The listing builds one solid part. Answer for the finished solid, in the listing's coordinates (mm). Face numbers are marked on the shaded views. A direction names the side the tool comes from. Round coordinates to 2 decimals unless told otherwise and drop trailing zeros. Order: outer loops, then holes, each group sorted by start corner. A loop starts at its lowest first (then second) coordinate and runs counter-clockwise, first axis right, second up. Notation, with made-up numbers: (51, -16) -> (81, -16) arc R24 cw to (81, 16) -> close; hole circle Ø10 at (63.25, -16.75). An arc over 180 degrees is marked (long way). Return JSON: item names as keys, results as strings. Group by question number.
(1) Determine the mould class of the marked faces 4, 5, 6 and 7 for opening direction Y: +Y half, -Y half, draft (parallel to the pull), parting line (faces both ways), or undercut.
(2) Consider line 1 (Y direction, x = -215.5, z = -3); line 2 (X direction, y = 70.5, z = -13.5); line 3 (Z direction, x = -154, y = 198.5). Determine where each line is inside the solid, lowest interval first. Write a range as [from, to].
(3) The part is cut by section D-D (x = 8.5). Determine the outline of the cut face in (y, z).
(4) Which of the six approach directions +Z, -Z, +X, -X, +Y, -Y give full straight-line access (tool end or side, diameter ignored) to the marked faces 1, 2 and 3?
(5) The part is cut by section A-A (y = 70). Determine the outline of the cut face in (x, z), plus the area to 3 significant figures.
(6) The part is cut by section C-C (z = 13). Determine the outline of the cut face in (x, y).
(7) The part is cut by section B-B (x = -176.5). Determine the outline of the cut face in (y, z), plus the area to 3 significant figures.
(8) Each of these flat-tipped pins is pushed along its axis until it touches: pin 1 (8 mm diameter, centred on y = 164, z = -6, fed in from +X); pin 2 (20.5 mm diameter, centred on x = -138, z = -11, fed in from -Y); pin 3 (1 mm diameter, centred on y = -27, z = -1, fed in from +X). Where does it stop, or does it pass through?
from build123d import *

# Parameters (mm, degrees)
F0_W     = 264.3314376473
F0_H     = 61.0694549978
F1_DEPTH = 229.87
F2_W     = 56.2751591206
F2_H     = 239.2987646163
F3_DEPTH = 64.008
F4_W     = 215.0589334778
F4_H     = 71.1349770427
F4_H_2   = 52.3396320641
F5_DEPTH = 25.4
F6_R     = 10.0158804511
F6_R_2   = 9.2218909308
F7_DEPTH = 42.926


with BuildPart() as f1:
    # F0 (on Right) → F1 (new body)
    with BuildSketch(Plane.YZ):
        with Locations((76.9639723003, -54.1143957525)):
            Rectangle(F0_W, F0_H)
    extrude(amount=-F1_DEPTH)

    # F2 (on face) → F3 (join)
    with BuildSketch(Plane.XY.offset(-23.5796682537)):
        with Locations((-249.6691197157, 71.1772423238)):
            Rectangle(F2_W, F2_H)
    extrude(amount=F3_DEPTH)

    # F4 (on face) → F5 (join)
    with BuildSketch(Plane.XY.offset(-23.5796682537)):
        with Locations((-114.0020734165, -7.937643677)):
            Rectangle(F4_W, F4_H)
        with Locations((-114.0020734165, 103.1337883323)):
            Rectangle(F4_W, F4_H_2)
    extrude(amount=F5_DEPTH)

    # F6 (on face) → F7 (join)
    with BuildSketch(Plane.YZ.offset(-6.4726066776)):
        with Locations((-20.9178049117, -11.1334202811)):
            Circle(F6_R)
        with Locations((102.3681536317, -10.6532974169)):
            Circle(F6_R_2)
    extrude(amount=F7_DEPTH)


solid = f1.part
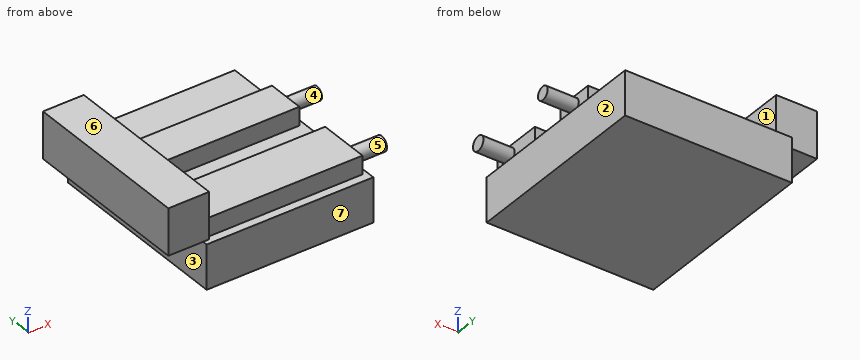
Answer below:
{
 "1": {"face 4": "undercut", "face 5": "undercut", "face 6": "draft", "face 7": "-Y half"},
 "2": {"line 1": "y = [-43.51, 27.63], [76.96, 129.3]", "line 2": "x = [-277.81, -221.53]", "line 3": "z = [-84.65, -23.58]"},
 "3": {"outline": "circle Ø20.03 at (-20.92, -11.13); circle Ø18.44 at (102.37, -10.65)"},
 "4": {"face 1": "+Z, +X", "face 2": "-Z, +X, +Y, -Y", "face 3": "-Z, -X, +Y, -Y"},
 "5": {"outline": "(-277.81, -23.58) -> (-229.87, -23.58) -> (-229.87, -84.65) -> (0, -84.65) -> (0, -23.58) -> (-221.53, -23.58) -> (-221.53, 40.43) -> (-277.81, 40.43) -> close", "area": "17,600 mm²"},
 "6": {"outline": "(-277.81, -48.47) -> (-221.53, -48.47) -> (-221.53, 190.83) -> (-277.81, 190.83) -> close"},
 "7": {"outline": "(-55.2, -84.65) -> (209.13, -84.65) -> (209.13, -23.58) -> (129.3, -23.58) -> (129.3, 1.82) -> (76.96, 1.82) -> (76.96, -23.58) -> (27.63, -23.58) -> (27.63, 1.82) -> (-43.51, 1.82) -> (-43.51, -23.58) -> (-55.2, -23.58) -> close", "area": "19,300 mm²"},
 "8": {"pin 1": "stops at x = -221.53", "pin 2": "stops at y = -43.51", "pin 3": "stops at x = -6.47"}
}
